from build123d import *

# Parameters (mm, degrees)
SCHIZZO1_W                   = 185
SCHIZZO1_H                   = 6
ESTRUSIONE_ESTRUSIONE1_DEPTH = 1.5
SCHIZZO2_OUTSIDE_W           = 224.02
SCHIZZO2_OUTSIDE_H           = 45.02
TAGLIO_ESTRUSIONE1_DEPTH     = 1.5
SCHIZZO5_W                   = 2.294465176
SCHIZZO5_H                   = 1.827727815
SCHIZZO5_R                   = 0.75
TAGLIO_ESTRUSIONE3_DEPTH     = 4.5
SCHIZZO6_R                   = 1.25
ESTRUSIONE_ESTRUSIONE3_DEPTH = 1.5
SCHIZZO7_R                   = 0.75
TAGLIO_ESTRUSIONE4_DEPTH     = 1.5


with BuildPart() as part:
    # Schizzo1 → Estrusione-Estrusione1 (new body)
    with BuildSketch(Plane.XY):
        with Locations((-92.5, 3)):
            Rectangle(SCHIZZO1_W, SCHIZZO1_H)
    extrude(amount=ESTRUSIONE_ESTRUSIONE1_DEPTH)

    # Schizzo2 outside → Taglio-Estrusione1 (cut)
    with BuildSketch(Plane.XY.offset(1.5)):
        with Locations((-92.5, 3)):
            Rectangle(SCHIZZO2_OUTSIDE_W, SCHIZZO2_OUTSIDE_H)
        with BuildLine():
            Line((-184.5, 0), (-184, 0))
            ThreePointArc((-184, 0), (-183.646446609, 0.146446609), (-183.5, 0.5))
            Line((-183.5, 0.5), (-183.5, 4))
            ThreePointArc((-183.5, 4), (-183.353553391, 4.353553391), (-183, 4.5))
            Line((-183, 4.5), (-160.5, 4.5))
            ThreePointArc((-160.5, 4.5), (-160.146446609, 4.353553391), (-160, 4))
            Line((-160, 4), (-160, 1.75))
            ThreePointArc((-160, 1.75), (-159.853553391, 1.396446609), (-159.5, 1.25))
            Line((-159.5, 1.25), (0, 1.25))
            Line((0, 1.25), (0, 2.75))
            Line((0, 2.75), (-158, 2.75))
            ThreePointArc((-158, 2.75), (-158.353553391, 2.896446609), (-158.5, 3.25))
            Line((-158.5, 3.25), (-158.5, 5.5))
            ThreePointArc((-158.5, 5.5), (-158.646446609, 5.853553391), (-159, 6))
            Line((-159, 6), (-184.5, 6))
            ThreePointArc((-184.5, 6), (-184.853553391, 5.853553391), (-185, 5.5))
            Line((-185, 5.5), (-185, 0.5))
            ThreePointArc((-185, 0.5), (-184.853553391, 0.146446609), (-184.5, 0))
        make_face(mode=Mode.SUBTRACT)
    extrude(amount=-TAGLIO_ESTRUSIONE1_DEPTH, mode=Mode.SUBTRACT)

    # Schizzo5 → Taglio-Estrusione3 (cut)
    with BuildSketch(Plane.XZ):
        with Locations((-184.019602527, 0.694189627)):
            Rectangle(SCHIZZO5_W, SCHIZZO5_H)
        with Locations(Location((-184.25, 0.75, 0), (0, 0, 180))):
            Circle(SCHIZZO5_R, mode=Mode.SUBTRACT)
    extrude(amount=-TAGLIO_ESTRUSIONE3_DEPTH, mode=Mode.SUBTRACT)

    # Schizzo6 → Estrusione-Estrusione3 (add)
    with BuildSketch(Plane(origin=(0, 2.75, 0), x_dir=(1, 0, 0), z_dir=(0, 1, 0))):
        with Locations((-1.224744871, -1.25)):
            Circle(SCHIZZO6_R)
    extrude(amount=-ESTRUSIONE_ESTRUSIONE3_DEPTH)

    # Schizzo7 → Taglio-Estrusione4 (cut)
    with BuildSketch(Plane(origin=(0, 2.75, 0), x_dir=(1, 0, 0), z_dir=(0, 1, 0))):
        with Locations(Location((-1.224744871, -1.25, 0), (0, 0, 270))):
            Circle(SCHIZZO7_R)
        with BuildLine():
            Line((-1.224744871, 0), (-1.224744871, 0.534346319))
            Line((-1.224744871, 0.534346319), (0.72573961, 0.534346319))
            Line((0.72573961, 0.534346319), (0.72573961, -1.25))
            Line((0.72573961, -1.25), (0.025255129, -1.25))
            ThreePointArc((0.025255129, -1.25), (-0.340861395, -0.366116524), (-1.224744871, 0))
        make_face()
    extrude(amount=-TAGLIO_ESTRUSIONE4_DEPTH, mode=Mode.SUBTRACT)


solid = part.part
Design review of the part built by this model. Coordinates are the model's own, in mm. A direction names the side the tool comes from. Coordinates: 2 decimals unless noted, no trailing zeros. Loops run counter-clockwise (first coordinate to the right, second up) from the corner with the lowest first, then second, coordinate; pieces in that order, holes last.
Item 1: Wall thickness on L1, parallel to X at y = 3.75, z = 0.7; L2, parallel to X at y = 1.9, z = 1.25; L3, parallel to Z at x = -126.5, y = 1.75: over which ranges is each line inside the solid? List them lowest first.
Completed:
L1: x = -185 to -183.5, -160 to -158.5
L2: x = -184.81 to -183.69, -160 to -1.97, -0.47 to 0.03
L3: z = 0 to 1.5
Item 2: Clearance check with flat-ended pins moving along their axes: pin 1 (0.8 mm diameter, centred on y = 3.5, z = 1, fed in from -X); pin 2 (1.5 mm diameter, centred on x = -71, y = 1, fed in from +Z); pin 3 (0.8 mm diameter, centred on x = -177.5, z = 0.5, fed in from -Y); pin 4 (0.8 mm diameter, centred on x = -84, z = 1, fed in from +Y). State where each tip first meets the part, or that it passes through.
Completed:
pin 1: stops at x = -185
pin 2: stops at z = 1.5
pin 3: stops at y = 4.5
pin 4: stops at y = 2.75
Item 3: For faces 1 (the flat face through (-94.15, 2.58, 1.5)), 2 (the flat face through (-93.54, 2.58, 0)), list the 3-axis set-ups (+Z, -Z, +X, -X, +Y, -Y) from which the entire face can be reached by the end or side of a thin tool; tool diameter is ignored.
Completed:
face 1: +Z, -X, +Y, -Y
face 2: -Z, +X, -X, +Y, -Y
Item 4: Add section A-A (x = -76). Write out the cut boundary in (y, z).
Completed:
outline: (1.25, 0) - (2.75, 0) - (2.75, 1.5) - (1.25, 1.5) - close
